```python
from build123d import *

# Parameters (mm, degrees)
F1_DEPTH = 172
F3_DEPTH = 10
F5_W     = 132
F5_H     = 10
F6_DEPTH = 35
F8_D     = 10


with BuildPart() as f1:
    # F0 (on Front) → F1 (new body)
    with BuildSketch(Plane.XZ):
        Polygon((-25, 0), (0, 0), (10, 0), (10, 17), (10, 60), (0, 60), (0, 17), (-25, 17), align=None)
    extrude(amount=F1_DEPTH)

    # F2 (on face) → F3 (cut)
    with BuildSketch(Plane(origin=(0, 0, 0), x_dir=(0, -1, 0), z_dir=(-1, 0, 0))):
        with BuildLine():
            Line((140, 31), (140, 60))
            Line((140, 60), (32, 60))
            Line((32, 60), (32, 31))
            ThreePointArc((32, 31), (33.464466, 27.464466), (37, 26))
            Line((37, 26), (135, 26))
            ThreePointArc((135, 26), (138.535534, 27.464466), (140, 31))
        make_face()
    extrude(amount=-F3_DEPTH, mode=Mode.SUBTRACT)

    # F5 (on offset) → F6 (cut)
    with BuildSketch(Plane.YZ.offset(-25)):
        with Locations((-86, 5)):
            Rectangle(F5_W, F5_H)
    extrude(amount=F6_DEPTH, mode=Mode.SUBTRACT)

    # F8 (through all)
    with Locations(Plane(origin=(0, 0, 0), x_dir=(0, -1, 0), z_dir=(-1, 0, 0))):
        with Locations((16, 48), (156, 48)):
            Hole(F8_D / 2)


solid = f1.part
```
Model file for the job. Use its own axes, mm. A direction names the side the tool comes from. Give positions to 0.01 mm unless a question says otherwise; leave off trailing zeros. Write each loop counter-clockwise with the first axis right and the second up, starting at its lowest first coordinate (ties: lowest second). Pieces come first, ordered by that corner, then holes. Notation, with made-up numbers: (8.25, 73) - (58.25, 73) arc R27 cw to (58.25, 96) - close; hole circle Ø7 at (27, 57). An arc over 180 degrees is marked (long way). One line per question, with ' | ' between items. Start each with the question number.
(1) Pin check, flat tips, straight feed: P1, Ø12, axis at x = -7, y = -56.5, coming from the +Z side; P2, Ø5, axis at x = 6, y = -77.5, coming from the +Z side; P3, Ø1.5, axis at x = -3.5, y = -141, coming from the -Z side; P4, Ø9, axis at y = -16, z = 48, coming from the -X side. Stop position of each tip, or through.
(2) Wall check: line 1 along Z through (x, y) = (3, -156); line 2 along Y through (x, z) = (5.5, 31); line 3 along Z through (x, y) = (-18, -52.5). Give the ranges that are in metal, low to high. Write a range as from..to.
(3) Slice it at C-C on z = 37. Write the cut outline in (x, y), plus the area to 3 significant figures.
(4) Slice it at D-D on x = 3.5. Write the cut outline in (y, z).
(5) Slice it at B-B on y = -16. Write the cut outline in (x, z).
(6) Two-plate mould, pull along Z, no slides. Class faces 5 (the face through (-8, -162, 0)), 6 (the face through (5, -85, 26)), 7 (the face through (5.07, -16.651, 52.957)), 8 (the face through (5, -160, 51)): +Z half, -Z half, draft (parallel to the pull), parting line (faces both ways), or undercut.
(7) Slice it at A-A on z = 48. Write the cut outline in (x, y).
(8) 3-axis set-ups, long thin cutter, end or side, ignore diameter. For faces 1 (the face through (4, -172, 24)), 2 (the face through (-8, -152, 5)), 3 (the face through (5, -32, 46)), 4 (the face through (-12, -85, 17)): which of +Z, -Z, +X, -X, +Y, -Y reach the whole face in a straight line?
Results below:
1) P1: z = 17 | P2: z = 26 | P3: z = 10 | P4: through
2) line 1: 0..43, 53..60 | line 2: -172..-140, -32..0 | line 3: 10..17
3) outline: (0, -172) - (10, -172) - (10, -140) - (0, -140) - close; (0, -32) - (10, -32) - (10, 0) - (0, 0) - close | area: 640 mm^2
4) outline: (-172, 0) - (-152, 0) - (-152, 10) - (-20, 10) - (-20, 0) - (0, 0) - (0, 60) - (-32, 60) - (-32, 31) arc R5 cw to (-37, 26) - (-135, 26) arc R5 cw to (-140, 31) - (-140, 60) - (-172, 60) - close; hole circle Ø10 at (-156, 48); hole circle Ø10 at (-16, 48)
5) outline: (-25, 0) - (10, 0) - (10, 43) - (0, 43) - (0, 17) - (-25, 17) - close; (0, 53) - (10, 53) - (10, 60) - (0, 60) - close
6) face 5: -Z half | face 6: +Z half | face 7: undercut | face 8: undercut
7) outline: (0, -172) - (10, -172) - (10, -161) - (0, -161) - close; (0, -151) - (10, -151) - (10, -140) - (0, -140) - close; (0, -32) - (10, -32) - (10, -21) - (0, -21) - close; (0, -11) - (10, -11) - (10, 0) - (0, 0) - close
8) face 1: +Z, -Z, +X, -X, -Y | face 2: -Z, +X, -X | face 3: +Z, +X, -X | face 4: +Z, -X, +Y, -Y
